Input: part model. Units: mm. Frame: model coordinates. A direction names the side the tool comes from. Coordinates: 2 decimals unless noted, no trailing zeros. Put each result on its own line as item: value. Start each with the question number.
1. Pull-direction query (Y, two-part tool) for faces 3 (the flat face through (31.166, 15.642, 0.986)), 4 (the flat face through (25, 27, 0)), 5 (the flat face through (23, 17.039, 1)), 6 (the flat face through (31.6, 19.956, 1)); classes: released by +Y, released by -Y, zero draft, split by the parting line, or undercut.
2. Access query for faces 1 (the flat face through (21, 11.206, 1)), 2 (the flat face through (13.49, 33.37, 0.99)). Directions: +Z, -Z, +X, -X, +Y, -Y. A direction counts if a zero-diameter tool reaches every point of the face in a straight line with its end or side. Return the directions, or none.
3. Line query: line 1 (Y direction, x = 22, z = 0.3); line 2 (X direction, y = 15, z = 1.85); line 3 (Y direction, x = 26, z = 1.75). Output: solid intervals per line, ascending.
4. Cut plane A-A, the plane x = 21. Count the separate pieces of the cut face and the enclosed holes in it, and give its area (3 significant figures).
5. Pin query (flat end, axial travel): pin 1 (1.5 mm diameter, centred on x = 23.5, y = 19, fed in from +Z); pin 2 (1 mm diameter, centred on x = 31.5, z = 1.5, fed in from +Y); pin 3 (1 mm diameter, centred on x = 23.5, z = 1.5, fed in from +Y); pin 4 (1 mm diameter, centred on x = 27.5, z = 0.5, fed in from +Y). Return the tip coordinate at first contact, or that it passes through.
from build123d import *

# Parameters (mm, degrees)
BOSS_EXTRU_1_DEPTH     = 2
D_GAGEMENT_M1_61_D     = 2.8
D_GAGEMENT_M1_61_DEPTH = 50


with BuildPart() as part:
    # Esquisse1 → Boss.-Extru.1 (new body)
    with BuildSketch(Plane.XY):
        with BuildLine():
            Line((30.179082722, 11.205600965), (12.542363972, 11.205600965))
            Line((12.542363972, 11.205600965), (12.542363972, 11.693882215))
            add(Edge.make_bspline(
                [(12.542363972, 11.693882215), (12.881136709, 12.088648819), (13.542742266, 12.85960749), (14.508452904, 13.992781588), (15.418047611, 15.079454653), (16.277439508, 16.114606131), (17.087274316, 17.097820692), (17.840140522, 18.035083149), (18.546233089, 18.920390025), (19.194803638, 19.760040209), (19.797304838, 20.547404882), (20.339194184, 21.2889747), (20.841948632, 21.973542972), (21.277716543, 22.6165006), (21.676531137, 23.203798306), (22.009071616, 23.748203678), (22.301606172, 24.237636856), (22.610004896, 24.824218938), (22.935697027, 25.52406999), (23.275867169, 26.35140879), (23.564495095, 27.174588864), (23.798493759, 27.994304476), (23.982029168, 28.80936221), (24.112052658, 29.618129528), (24.193983215, 30.422653355), (24.204021871, 30.958014733), (24.209030639, 31.225132215)],
                knots=[0, 0, 0, 0, 0.0015606, 0.003047771, 0.004466519, 0.005811909, 0.007083975, 0.008287821, 0.009418461, 0.010481096, 0.011470701, 0.012392609, 0.013236481, 0.014018408, 0.014722618, 0.015365799, 0.015931906, 0.016432828, 0.017353171, 0.018246618, 0.019115508, 0.019968646, 0.020802615, 0.02162034, 0.022424923, 0.023226128, 0.023226128, 0.023226128, 0.023226128], degree=3))
            add(Edge.make_bspline(
                [(24.209030639, 31.225132215), (24.206655253, 31.414235122), (24.201968183, 31.787369618), (24.12375386, 32.332982208), (24.019318572, 32.858426919), (23.85158693, 33.35310546), (23.651423788, 33.825766135), (23.401285376, 34.273895228), (23.100563635, 34.693869832), (22.765183813, 35.090463219), (22.394783522, 35.445944183), (22.002313346, 35.762683678), (21.587212745, 36.028401492), (21.150868718, 36.246817438), (20.697063898, 36.416097723), (20.220705812, 36.533298704), (19.725615517, 36.606433615), (19.387236699, 36.616937759), (19.215541055, 36.622267631)],
                knots=[0, 0, 0, 0, 0.000566743, 0.001118287, 0.00165075, 0.002171624, 0.002681976, 0.00318912, 0.003707547, 0.004229397, 0.004745078, 0.005245322, 0.005740156, 0.006220562, 0.006706711, 0.007189888, 0.007689835, 0.008204817, 0.008204817, 0.008204817, 0.008204817], degree=3))
            add(Edge.make_bspline(
                [(19.215541055, 36.622267631), (18.936844993, 36.61344576), (18.389653493, 36.59612491), (17.597649359, 36.424792239), (16.849444788, 36.166203908), (16.151829751, 35.788732099), (15.506339966, 35.302359066), (14.907144288, 34.713738884), (14.356945555, 34.020964188), (14.04878719, 33.499173505), (13.890020222, 33.230340548)],
                knots=[0, 0, 0, 0, 0.000834959, 0.001639358, 0.002419767, 0.003203319, 0.004008008, 0.0048367, 0.00571722, 0.006653, 0.006653, 0.006653, 0.006653], degree=3))
            Line((13.890020222, 33.230340548), (13.076218139, 33.516798881))
            add(Edge.make_bspline(
                [(13.076218139, 33.516798881), (13.179054061, 33.852146444), (13.379157113, 34.504681753), (13.730639084, 35.441767759), (14.128497083, 36.308808373), (14.563282581, 37.10954717), (15.033600596, 37.844258143), (15.5420578, 38.513613494), (16.095126829, 39.111498004), (16.684071503, 39.642688482), (17.305618092, 40.104990045), (17.951897427, 40.51064322), (18.622014238, 40.85644043), (19.314800196, 41.13819172), (20.03030182, 41.35294052), (20.767979453, 41.510881359), (21.530961248, 41.602061284), (22.047337974, 41.615489489), (22.307988972, 41.622267631)],
                knots=[0, 0, 0, 0, 0.001052132, 0.00204729, 0.002999904, 0.003911781, 0.00477862, 0.005614594, 0.006430061, 0.00721836, 0.007990496, 0.00875099, 0.009505131, 0.010249855, 0.0109913, 0.011743387, 0.01251054, 0.013292467, 0.013292467, 0.013292467, 0.013292467], degree=3))
            add(Edge.make_bspline(
                [(22.307988972, 41.622267631), (22.679896981, 41.609915738), (23.413788868, 41.585541555), (24.487860289, 41.38745513), (25.508615399, 41.050279213), (26.468407849, 40.589262885), (27.355163704, 40.016933082), (28.150058294, 39.34282648), (28.841028925, 38.567355524), (29.408352915, 37.708211361), (29.86607553, 36.82218061), (30.202107309, 35.945268221), (30.419693518, 35.09420366), (30.446199504, 34.531420793), (30.459030639, 34.258986381)],
                knots=[0, 0, 0, 0, 0.001115183, 0.002200609, 0.003262944, 0.004331625, 0.005386232, 0.006420753, 0.00744909, 0.00849096, 0.009501334, 0.010434779, 0.011304864, 0.012121266, 0.012121266, 0.012121266, 0.012121266], degree=3))
            add(Edge.make_bspline(
                [(30.459030639, 34.258986381), (30.440330645, 33.771334999), (30.402419871, 32.782712091), (30.083359411, 31.300391879), (29.583549933, 29.80452581), (29.108010723, 28.841647649), (28.863978555, 28.347528048)],
                knots=[0, 0, 0, 0, 0.001461599, 0.002963122, 0.004529862, 0.006181366, 0.006181366, 0.006181366, 0.006181366], degree=3))
            add(Edge.make_bspline(
                [(28.863978555, 28.347528048), (28.76786982, 28.173010661), (28.56975854, 27.813273711), (28.23120618, 27.272143019), (27.865011588, 26.69861719), (27.444510098, 26.107661003), (26.987928456, 25.491384116), (26.501286537, 24.840310245), (25.957900083, 24.177108889), (25.388470702, 23.477928873), (24.771397811, 22.759712277), (24.117625487, 22.015788636), (23.425278319, 21.243370208), (22.689052157, 20.449438203), (21.91022666, 19.633010142), (21.091622049, 18.791368662), (20.243257466, 17.916656162), (19.65289757, 17.335092583), (19.352259805, 17.038934298)],
                knots=[0, 0, 0, 0, 0.000597577, 0.0012318, 0.001914401, 0.002638697, 0.003406954, 0.004215557, 0.005076755, 0.005978701, 0.006920711, 0.007917166, 0.008949842, 0.010032472, 0.011165284, 0.012334734, 0.013554755, 0.014820742, 0.014820742, 0.014820742, 0.014820742], degree=3))
            Line((19.352259805, 17.038934298), (25.745488972, 17.038934298))
            add(Edge.make_bspline(
                [(25.745488972, 17.038934298), (25.934313645, 17.037464211), (26.292485048, 17.034675682), (26.804467082, 17.053384982), (27.26500093, 17.059893125), (27.672690984, 17.089906602), (28.028799564, 17.114582451), (28.333895654, 17.142780825), (28.587044708, 17.1909813), (28.967040392, 17.271944811), (29.453325738, 17.483845597), (29.924483141, 17.844652989), (30.250271084, 18.262660952), (30.531456746, 18.706877056), (30.850559761, 19.283215692), (31.060390484, 19.717842386), (31.175176472, 19.955600965)],
                knots=[0, 0, 0, 0, 0.000566406, 0.001074386, 0.001536809, 0.001947791, 0.002300316, 0.002608033, 0.002865996, 0.003072901, 0.003773035, 0.00443598, 0.00482947, 0.005356773, 0.006012518, 0.006804464, 0.006804464, 0.006804464, 0.006804464], degree=3))
            Line((31.175176472, 19.955600965), (32.125697305, 19.955600965))
            Line((32.125697305, 19.955600965), (30.179082722, 11.205600965))
        make_face()
    extrude(amount=BOSS_EXTRU_1_DEPTH)

    # Dégagement M1.61
    with Locations(Plane.XY.offset(2)):
        with Locations((21.360723347, 13.792257827)):
            Hole(D_GAGEMENT_M1_61_D / 2, depth=D_GAGEMENT_M1_61_DEPTH)


solid = part.part
Report:
1. face 3: released by -Y
1. face 4: zero draft
1. face 5: undercut
1. face 6: released by +Y
2. face 1: +Z, -Z, +X, -X, -Y
2. face 2: +Z, -Z, -X
3. line 1: y = 11.21 to 12.55, 15.04 to 17.04, 19.73 to 23.74, 35.75 to 41.61
3. line 2: x = 15.35 to 20.65, 22.07 to 31.02
3. line 3: y = 11.21 to 17.04, 24.23 to 40.81
4. separate pieces: 4
4. enclosed holes: 0
4. area: 23.7 mm^2
5. pin 1: passes through
5. pin 2: stops at y = 19.96
5. pin 3: stops at y = 41.59
5. pin 4: stops at y = 40.24
